from build123d import *

# Parameters (mm, degrees)
F0_W       = 166.1031842232
F0_H       = 90.2919918299
F1_DEPTH   = 104.394
F1_FACE1_W = 166.1031842232
F1_FACE1_H = 104.394
F3_DEPTH   = 25.4
F5_DEPTH   = 306.324
F7_DEPTH   = 25.4
F8_R       = 12.9217505793
F9_DEPTH   = 104.395


# Not quite as in the source:
# - a pattern or mirror of a feature is missing from the dataset's text; its kind, count and spacing are read off the source's solid


with BuildPart() as f1:
    # F0 (on Top) → F1 (new body)
    with BuildSketch(Plane.XY):
        Rectangle(F0_W, F0_H)
    extrude(amount=F1_DEPTH)

    # F2 (on face) + F1_face1 (on face) → F3 (join)
    with BuildSketch(Plane(origin=(0, 45.1459959149, 0), x_dir=(-1, 0, 0), z_dir=(0, 1, 0))):
        with BuildLine():
            Line((28.1535676802, 104.394), (17.0834749636, 104.394))
            ThreePointArc((17.0834749636, 104.394), (0, 87.3105250364), (-17.0834749636, 104.394))
            Line((-17.0834749636, 104.394), (-28.1535676802, 104.394))
            ThreePointArc((-28.1535676802, 104.394), (0, 76.2404323198), (28.1535676802, 104.394))
        make_face()
    with BuildSketch(Plane(origin=(0, -45.1459959149, 52.197), x_dir=(1, 0, 0), z_dir=(0, -1, 0))):
        Rectangle(F1_FACE1_W, F1_FACE1_H)
    extrude(amount=F3_DEPTH, dir=(0, 1, 0))

    # F4 (on face) → F5 (cut)
    with BuildSketch(Plane(origin=(0, 45.1459959149, 0), x_dir=(-1, 0, 0), z_dir=(0, 1, 0))):
        with BuildLine():
            Line((17.0834749636, 104.394), (-17.0834749636, 104.394))
            ThreePointArc((-17.0834749636, 104.394), (0, 87.3105250364), (17.0834749636, 104.394))
        make_face()
    extrude(amount=-F5_DEPTH, mode=Mode.SUBTRACT)

    # F6 (on face) → F7 (join)
    with BuildSketch(Plane.XZ.offset(45.1459959149)):
        with BuildLine():
            ThreePointArc((-27.8307711085, 104.394), (0, 76.5632288915), (27.8307711085, 104.394))
            Line((27.8307711085, 104.394), (17.0834749636, 104.394))
            ThreePointArc((17.0834749636, 104.394), (0, 87.3105250364), (-17.0834749636, 104.394))
            Line((-17.0834749636, 104.394), (-27.8307711085, 104.394))
        make_face()
    extrude(amount=F7_DEPTH)

    # F8 (on face) → F9 (cut, through all)
    with BuildSketch(Plane.XY.offset(104.394)):
        with Locations((37.7448610961, 0)):
            Circle(F8_R)
    f9 = extrude(amount=-F9_DEPTH, mode=Mode.SUBTRACT)

    # F9_copies: F9 across plane
    add(f9.mirror(Plane(origin=(0, 0, 0), x_dir=(0, 0, -1), z_dir=(-1, 0, 0))), mode=Mode.SUBTRACT)


solid = f1.part
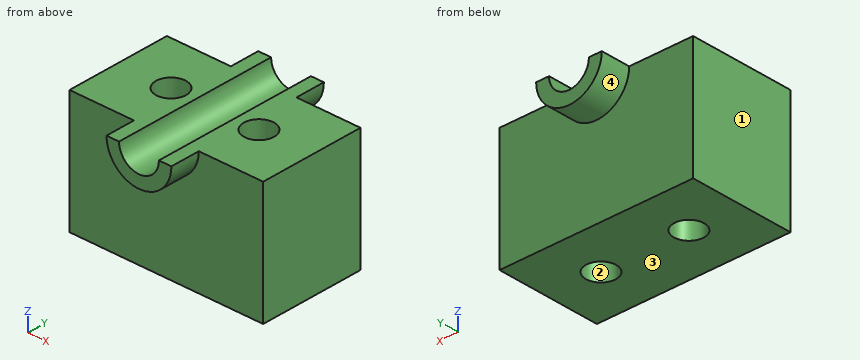
The listing builds one solid part. Answer for the finished solid, in the listing's coordinates (mm). Face numbers are marked on the shaded views. Give positions to 0.01 mm unless a question says otherwise; leave off trailing zeros. Write each loop counter-clockwise with the first axis right and the second up, starting at its lowest first coordinate (ties: lowest second). Pieces come first, ordered by that corner, then holes.
1) Find the intervals of material crossed by L1, parallel to X at y = -1, z = 70.5; L2, parallel to X at y = -9, z = 36; L3, parallel to Y at x = 33, z = 23, in increasing order.
2) Section A-A (y = 0) is taken. Write down the section's boundary in (x, z), and give its area (3 significant figures).
3) Section B-B (z = 48) is taken. Write down the section's boundary in (x, y).
4) Given P1, Ø6, axis at x = 4.5, y = 28.5, coming from the +Z side; P2, Ø8, axis at x = 50, y = 16.5, coming from the -Z side; P3, Ø15.5, axis at x = 37.74, y = 0, coming from the +Z side; P4, Ø3, axis at x = -61.5, z = 84, coming from the -Y side, each flat-ended and moving along its own axis, determine where each tip first touches the part or whether it passes through.
5) Section D-D (y = 24) is taken. Write down the section's boundary in (x, z), and give its area (3 significant figures).
6) Section C-C (x = -38) is taken. Write down the section's boundary in (y, z).
7) For a pull along X with two mould halves and no side action, classify the marked faces 1, 2, 3 and 4 as pulls with the +X half, pulls with the -X half, needs draft (parallel to the pull), parting line crosses it, or undercut.
Response:
1. L1: x = -83.05 to -50.63, -24.86 to 24.86, 50.63 to 83.05
1. L2: x = -83.05 to -47.02, -28.47 to 28.47, 47.02 to 83.05
1. L3: y = -45.15 to -12.02, 12.02 to 45.15
2. outline: (-83.05, 0) - (-50.67, 0) - (-50.67, 104.39) - (-83.05, 104.39) - close; (-24.82, 0) - (24.82, 0) - (24.82, 104.39) - (17.08, 104.39) arc R17.08 cw to (-17.08, 104.39) - (-24.82, 104.39) - close; (50.67, 0) - (83.05, 0) - (83.05, 104.39) - (50.67, 104.39) - close
2. area: 11,500 mm2
3. outline: (-83.05, -45.15) - (83.05, -45.15) - (83.05, 45.15) - (-83.05, 45.15) - close; hole circle Ø25.84 at (-37.74, 0); hole circle Ø25.84 at (37.74, 0)
4. P1: stops at z = 89.04
4. P2: stops at z = 0
4. P3: passes through
4. P4: stops at y = -45.15
5. outline: (-83.05, 0) - (83.05, 0) - (83.05, 104.39) - (17.08, 104.39) arc R17.08 cw to (-17.08, 104.39) - (-83.05, 104.39) - close
5. area: 16,900 mm2
6. outline: (-45.15, 0) - (-12.92, 0) - (-12.92, 104.39) - (-45.15, 104.39) - close; (12.92, 0) - (45.15, 0) - (45.15, 104.39) - (12.92, 104.39) - close
7. face 1: pulls with the -X half
7. face 2: undercut
7. face 3: needs draft
7. face 4: parting line crosses it
